```python
from build123d import *

# Parameters (mm, degrees)
F1_DEPTH = 20
F3_D     = 5
F3_DEPTH = 10
F3_TIP   = 1.5021515476
F4_D     = 5
F4_DEPTH = 10
F4_TIP   = 1.5021515476


with BuildPart() as f1:
    # F0 (on Right) → F1 (new body)
    with BuildSketch(Plane.YZ):
        with BuildLine():
            Line((-56.3612431288, 114.1744827852), (-56.3612431288, 14.1744827852))
            Line((-56.3612431288, 14.1744827852), (-6.3612431288, 14.1744827852))
            Line((-6.3612431288, 14.1744827852), (-6.3612431288, 114.1744827852))
            Line((-6.3612431288, 114.1744827852), (-13.8612431288, 114.1744827852))
            ThreePointArc((-13.8612431288, 114.1744827852), (-31.3612431288, 96.6744827852), (-48.8612431288, 114.1744827852))
            Line((-48.8612431288, 114.1744827852), (-56.3612431288, 114.1744827852))
        make_face()
    extrude(amount=F1_DEPTH)

    # F3
    with Locations(Plane(origin=(0, 0, 14.1744827852), x_dir=(1, 0, 0), z_dir=(0, 0, -1))):
        with Locations((10, 43.8612431288)):
            Hole(F3_D / 2, depth=F3_DEPTH)
            with Locations((0, 0, -(F3_DEPTH + F3_TIP / 2))):  # 118° drill point
                Cone(0, F3_D / 2, F3_TIP, mode=Mode.SUBTRACT)

    # F4
    with Locations(Plane(origin=(0, 0, 14.1744827852), x_dir=(1, 0, 0), z_dir=(0, 0, -1))):
        with Locations((10, 18.8612431288)):
            Hole(F4_D / 2, depth=F4_DEPTH)
            with Locations((0, 0, -(F4_DEPTH + F4_TIP / 2))):  # 118° drill point
                Cone(0, F4_D / 2, F4_TIP, mode=Mode.SUBTRACT)


solid = f1.part
```
Here's how the part is built. I have some questions about the finished solid (model axes, mm). A direction names the side the tool comes from. Coordinates: 2 decimals unless noted, no trailing zeros. Write each loop counter-clockwise with the first axis right and the second up, starting at its lowest first coordinate (ties: lowest second). Pieces come first, ordered by that corner, then holes. Notation, with made-up numbers: (5, 27) - (24, 27) arc R16 cw to (24, 32) - close; hole circle Ø6 at (23, -36). An arc over 180 degrees is marked (long way). One line per item, written item: value.
1) We'd pull the mould along X, two halves only. Please class faces 1 (the flat face through (10, -56.361, 65)), 2 (the cylindrical face through (10.33, -21.34, 19.24)), 3 (the flat face through (0, -32, 65)): pulls with the +X half, pulls with the -X half, needs draft (parallel to the pull), parting line crosses it, or undercut.
Model answer:
face 1: needs draft
face 2: undercut
face 3: pulls with the -X half
2) I'm going to push a flat-ended pin straight in: P1, Ø3, axis at x = 10, y = -18.86, coming from the -Z side. Where does the tip first touch, or does it pass through?
Model answer:
P1: stops at z = 24.77
3) On a 3-axis mill with a long thin cutter (end or side, diameter ignored), from which of +Z, -Z, +X, -X, +Y, -Y can I reach the whole of each face in a straight line? I mean faces 4 (the cylindrical face through (11.843, -45.551, 19.244)), 5 (the flat face through (10, -10, 114.174)). Say none if no direction works.
Model answer:
face 4: -Z
face 5: +Z, +X, -X, +Y, -Y
4) I need wall thicknesses on line 1 along Y through (x, z) = (10, 17.5); line 2 along Z through (x, y) = (17.25, -43.5); line 3 along Z through (x, y) = (7.5, -16.5). Which ranges of each line are inside material? Lowest first, please.
Model answer:
line 1: y = -56.36 to -46.36, -41.36 to -21.36, -16.36 to -6.36
line 2: z = 14.17 to 101.57
line 3: z = 14.17 to 104.93
5) Suppose I cut it at A-A on x = 5. Write out the boundary of the cut face in (y, z), and give its area (3 significant figures).
Model answer:
outline: (-56.36, 14.17) - (-6.36, 14.17) - (-6.36, 114.17) - (-13.86, 114.17) arc R17.5 cw to (-48.86, 114.17) - (-56.36, 114.17) - close
area: 4,520 mm²
